Verification items for the finished model (mm, model axes). A direction names the side the tool comes from. Give positions to 0.01 mm unless a question says otherwise; leave off trailing zeros. Loops run counter-clockwise (first coordinate to the right, second up) from the corner with the lowest first, then second, coordinate; pieces in that order, holes last. Notation, with made-up numbers: (65, -1) - (90, -1) arc R27 cw to (90, 17) - close; hole circle Ø3 at (4, 87.5). An arc over 180 degrees is marked (long way). Answer in a Markdown table with one row per item.
```python
from build123d import *

# Parameters (mm, degrees)
BOSS_EXTRUDE1_DEPTH = 25.4


with BuildPart() as part:
    # Sketch2 → Boss-Extrude1 (new body)
    with BuildSketch(Plane.XY):
        with BuildLine():
            Line((-157.342145667, -6.429422494), (-157.342145667, -40.465422494))
            ThreePointArc((-157.342145667, -40.465422494), (-141.629836885, -59.2207502), (-120.41171865, -47.037547699))
            ThreePointArc((-120.41171865, -47.037547699), (-82.973266833, 2.473921311), (-24.309833539, 22.762460739))
            ThreePointArc((-24.309833539, 22.762460739), (-14.196167577, 21.07351252), (-5.57436841, 15.523434648))
            ThreePointArc((-5.57436841, 15.523434648), (23.363587608, 18.205213028), (15.981707982, 46.314021024))
            ThreePointArc((15.981707982, 46.314021024), (14.448779168, 46.900655432), (12.909621311, 47.470746453))
            ThreePointArc((12.909621311, 47.470746453), (-76.05269782, 52.166250257), (-152.440538162, 6.326967661))
            ThreePointArc((-152.440538162, 6.326967661), (-156.074572062, 0.403425483), (-157.342145667, -6.429422494))
        make_face()
        with BuildLine():
            Line((-147.944145667, -40.465422494), (-147.944145667, -6.429422494))
            ThreePointArc((-147.944145667, -6.429422494), (-138.292145667, 3.222577506), (-128.640145667, -6.429422494))
            Line((-128.640145667, -6.429422494), (-128.640145667, -40.465422494))
            ThreePointArc((-128.640145667, -40.465422494), (-138.292145667, -50.117422494), (-147.944145667, -40.465422494))
        make_face(mode=Mode.SUBTRACT)
    extrude(amount=BOSS_EXTRUDE1_DEPTH)


solid = part.part
```
Q1. Draft check along Y on faces 4 (the face through (-147.944, -24, 13)), 5 (the face through (-142, -59.15, 12.52)), 6 (the face through (-87, 12, 0)). Enter one of: +Y half, -Y half, draft (parallel to the pull), parting line (faces both ways), or undercut.
Completed:
| item | result |
|---|---|
| face 4 | undercut |
| face 5 | -Y half |
| face 6 | draft |
Q2. Tool access check on faces 1 (the face through (-87, 12, 25.4)), 2 (the face through (-138.5, 3.22, 12.52)), 3 (the face through (-83.685, 1.953, 12.522)). Record the directions out of +Z, -Z, +X, -X, +Y, -Y that give a thin tool (end or side, any length) a straight path to the whole face; none if there is none.
Completed:
| item | result |
|---|---|
| face 1 | +Z, +X, -X, +Y, -Y |
| face 2 | +Z, -Z |
| face 3 | +Z, -Z, -Y |
Q3. Sectioned sample at A-A (y = -31). Record the cut outline in (x, z), and give its area (3 significant figures).
Completed:
| item | result |
|---|---|
| outline | (-157.34, 0) - (-147.94, 0) - (-147.94, 25.4) - (-157.34, 25.4) - close; (-128.64, 0) - (-112.95, 0) - (-112.95, 25.4) - (-128.64, 25.4) - close |
| area | 637 mm^2 |
Q4. Go/stop test with flat-tipped pins: P1, Ø8, axis at x = -89.5, z = 14.5, coming from the +Y side; P2, Ø5, axis at y = -26.5, z = 17, coming from the +X side; P3, Ø12.5, axis at y = -15.5, z = 9, coming from the +X side. Record where each tip stops, or that it passes through.
Completed:
| item | result |
|---|---|
| P1 | y = 49.49 |
| P2 | x = -108.6 |
| P3 | x = -96.55 |
Q5. Sectioned sample at D-D (x = -26.5). Record the cut outline in (y, z), and give its area (3 significant figures).
Completed:
| item | result |
|---|---|
| outline | (22.66, 0) - (56.14, 0) - (56.14, 25.4) - (22.66, 25.4) - close |
| area | 850 mm^2 |
Q6. Sectioned sample at B-B (z = 14). Record the cut outline in (x, y).
Completed:
| item | result |
|---|---|
| outline | (-157.34, -40.47) arc R19.05 ccw to (-120.41, -47.04) arc R106.68 cw to (-24.31, 22.76) arc R25.4 cw to (-5.57, 15.52) arc R19.05 ccw (long way) to (15.98, 46.31) arc R152.4 ccw to (12.91, 47.47) arc R152.4 ccw to (-152.44, 6.33) arc R19.05 ccw to (-157.34, -6.43) - close; hole (-147.94, -40.47) arc R9.65 ccw to (-128.64, -40.47) - (-128.64, -6.43) arc R9.65 ccw to (-147.94, -6.43) - close |
Q7. Sectioned sample at C-C (y = 18). Record the cut outline in (x, z), and give its area (3 significant figures).
Completed:
| item | result |
|---|---|
| outline | (-140.71, 0) - (-52.05, 0) - (-52.05, 25.4) - (-140.71, 25.4) - close; (-8.52, 0) - (23.22, 0) - (23.22, 25.4) - (-8.52, 25.4) - close |
| area | 3,060 mm^2 |
Q8. Thickness scan on line 1 (X direction, y = -12, z = 21.5); line 2 (Y direction, x = -138.5, z = 15); line 3 (X direction, y = 14, z = 2.25). Record the ranges inside material, lowest first.
Completed:
| item | result |
|---|---|
| line 1 | -157.34 to -147.94, -128.64 to -99.14 |
| line 2 | -59.51 to -50.12, 3.22 to 19.93 |
| line 3 | -145.02 to -62.8, -3.82 to 19.33 |
